from build123d import *

# Parameters (mm, degrees)
F1_DEPTH = 4
F2_R     = 2
F2_R_2   = 3
F3_DEPTH = 25
F4_R     = 4.99999


# Not quite as in the source:
# - a fillet or chamfer is up to 0.001 mm smaller than in the source, because OpenCascade refuses the exact size


with BuildPart() as f1:
    # F0 (on Top) → F1 (new body)
    with BuildSketch(Plane.XY):
        Polygon((-20, 14), (-20, 0), (20, 0), (20, 14), (5, 14), (5, 79), (-5, 79), (-5, 14), align=None)
    extrude(amount=F1_DEPTH)

    # F2 (on Top) → F3 (cut)
    with BuildSketch(Plane.XY):
        with Locations((-15, 7.5)):
            Circle(F2_R)
        with Locations((15, 7.5)):
            Circle(F2_R)
        with Locations((0, 75)):
            Circle(F2_R)
        with Locations((0, 7.5)):
            Circle(F2_R_2)
    extrude(amount=F3_DEPTH, mode=Mode.SUBTRACT)

    # F4 (radius 5 in the source; OpenCascade refuses exactly that, so slightly less here)
    f4_edges = [f1.edges().sort_by_distance(p)[0] for p in [
        (-5, 79, 2),
        (5, 79, 2),
        (20, 0, 2),
        (-20, 0, 2),
        (-20, 14, 2),
        (20, 14, 2),
        (5, 14, 2),
        (-5, 14, 2),
    ]]
    fillet(f4_edges, radius=F4_R)


solid = f1.part
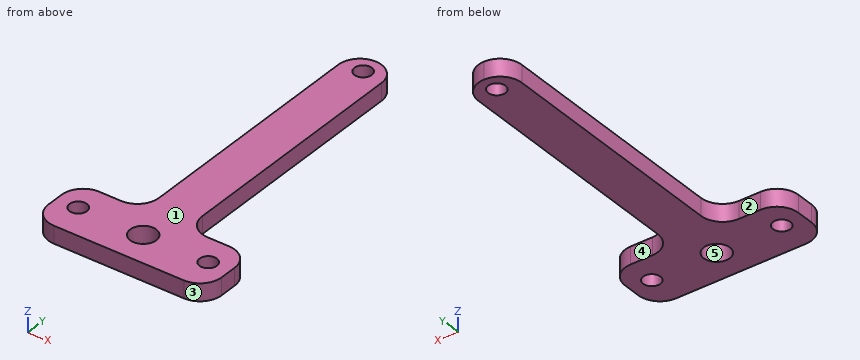
Here's how the part is built. I have some questions about the finished solid (model axes, mm). Face numbers are marked on the shaded views. A direction names the side the tool comes from. Round coordinates to 2 decimals unless told otherwise and drop trailing zeros. Order: outer loops, then holes, each group sorted by start corner. A loop starts at its lowest first (then second) coordinate and runs counter-clockwise, first axis right, second up. Notation, with made-up numbers: M 31.25,42.25 L 40.25,42.25 A24 ccw 40.25,52.25 Z; hole C -22.75,58 d6. An arc over 180 degrees is marked long. One line per question, with ' | ' between items.
1) Imagine slicing it at B-B, the plane y = 75. Write out the boundary of the cut face in (x, z), plus the area to 3 significant figures.
Checked values:
outline: M -4.9,0 L -2,0 L -2,4 L -4.9,4 Z; M 2,0 L 4.9,0 L 4.9,4 L 2,4 Z | area: 23.2 mm²
2) We'd pull the mould along X, two halves only. Please class the marked faces 3, 4 and 5: released by +X, released by -X, zero draft, split by the parting line, or undercut.
Checked values:
face 3: released by +X | face 4: zero draft | face 5: undercut
3) Imagine slicing it at A-A, the plane z = 1.75. Count the separate pieces of the cut face and the enclosed holes in it, plus the area to 3 significant figures.
Checked values:
separate pieces: 1 | enclosed holes: 4 | area: 1,120 mm²
4) I'm going to push flat-ended pins straight in: pin 1 Ø12 at (x, y) = (13, 32.5) entering from +Z; pin 2 Ø2 at (x, z) = (-13.5, 2) entering from +Y; pin 3 Ø2 at (x, z) = (3, 2.5) entering from +Y; pin 4 Ø1.5 at (y, z) = (38, 2.5) entering from -X. Where does each tip first touch, or does it pass through?
Checked values:
pin 1: passes through | pin 2: stops at y = 14 | pin 3: stops at y = 78.58 | pin 4: stops at x = -5
5) Imagine slicing it at C-C, the plane x = -6. Write out the boundary of the cut face in (y, z).
Checked values:
outline: M 0,0 L 16,0 L 16,4 L 0,4 Z
6) I need wall thicknesses on line 1 (Y direction, x = 0, z = 1.4); line 2 (X direction, y = 7.5, z = 0.95); line 3 (Y direction, x = 15, z = 2.7). Which ranges of each line are inside material? Lowest first, please.
Checked values:
line 1: y = 0 to 4.5, 10.5 to 73, 77 to 79 | line 2: x = -20 to -17, -13 to -3, 3 to 13, 17 to 20 | line 3: y = 0 to 5.5, 9.5 to 14
7) On a 3-axis mill with a long thin cutter (end or side, diameter ignored), from which of +Z, -Z, +X, -X, +Y, -Y can I reach the whole of each face in a straight line? I mean the marked faces 1 and 2. Say none if no direction works.
Checked values:
face 1: +Z, +X, -X, +Y, -Y | face 2: +Z, -Z, -X, +Y
